Check sheet for the drawn part. Datum: minimum x, y, z corner. Units: mm. A direction names the side the tool comes from. Round coordinates to 2 decimals unless told otherwise and drop trailing zeros. Order: outer loops, then holes, each group sorted by start corner. A loop starts at its lowest first (then second) coordinate and runs counter-clockwise, first axis right, second up. Notation, with made-up numbers: (58, -34) -> (82, -34) arc R33 cw to (82, -5) -> close; hole circle Ø11 at (-2.5, -32). An arc over 180 degrees is marked (long way). Answer in a Markdown table with one row per item.
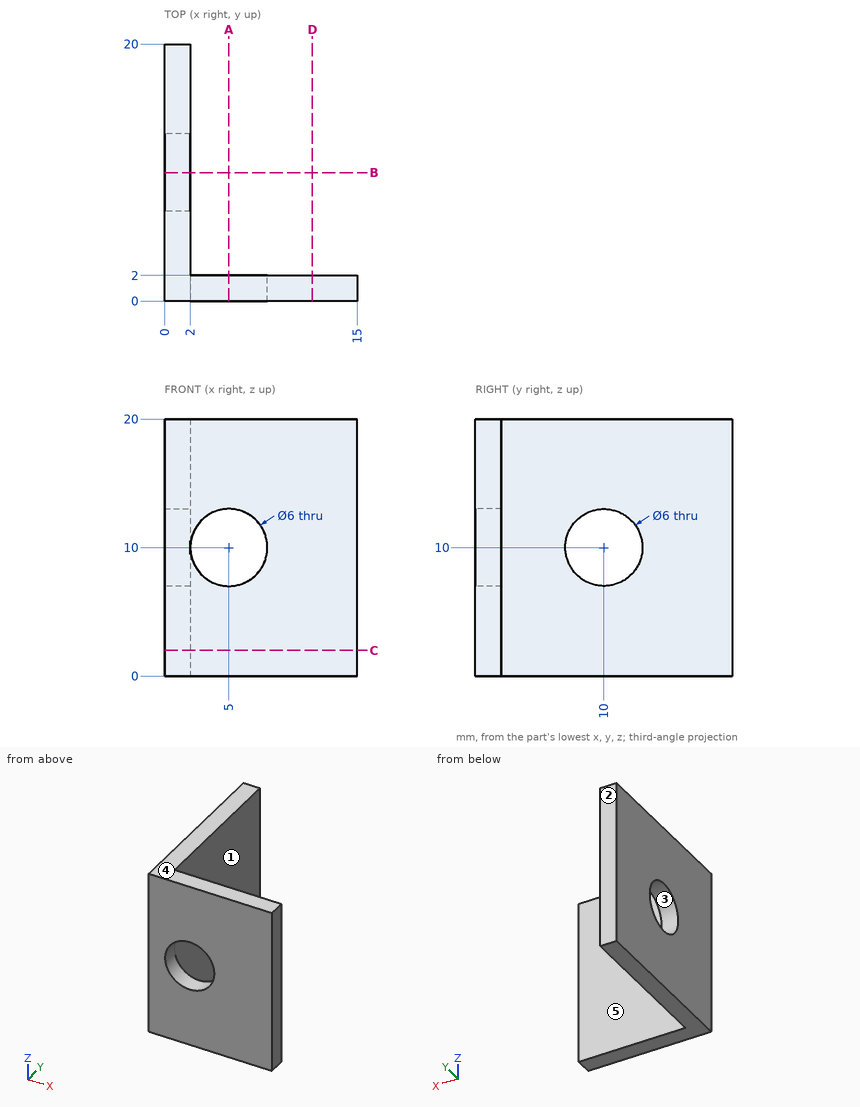
(1) Depth check by flat-ended pin: pin 1 Ø3.5 at (x, z) = (5, 10) entering from +Y; pin 2 Ø8 at (y, z) = (16.5, 12) entering from +X; pin 3 Ø4 at (x, y) = (12.5, 2.5) entering from -Z; pin 4 Ø6.5 at (x, z) = (7.5, 10) entering from +Y. Enter the tip coordinate at first touch or a pass-through.
Solutions:
| item | result |
|---|---|
| pin 1 | through |
| pin 2 | x = 2 |
| pin 3 | z = 0 |
| pin 4 | y = 2 |
(2) Section check C-C on z = 2. Record the boundary of the cut face in (x, y).
Solutions:
| item | result |
|---|---|
| outline | (0, 0) -> (15, 0) -> (15, 2) -> (2, 2) -> (2, 20) -> (0, 20) -> close |
(3) Scan lines: probe 1 along X at (y, z) = (0.5, 10); probe 2 along Z at (x, y) = (5, 1.3). Record each from-to range of solid material in increasing order. Write a range as from..to.
Solutions:
| item | result |
|---|---|
| probe 1 | 0..2, 8..15 |
| probe 2 | 0..7, 13..20 |
(4) Draft check along Y on the marked faces 3, 4 and 5. Enter one of: pulls with the +Y half, pulls with the -Y half, needs draft (parallel to the pull), parting line crosses it, or undercut.
Solutions:
| item | result |
|---|---|
| face 3 | undercut |
| face 4 | needs draft |
| face 5 | pulls with the +Y half |
(5) Section check D-D on x = 11.5. Record the boundary of the cut face in (y, z), plus the area to 3 significant figures.
Solutions:
| item | result |
|---|---|
| outline | (0, 0) -> (2, 0) -> (2, 20) -> (0, 20) -> close |
| area | 40.0 mm^2 |
(6) Section check A-A on x = 5. Record the boundary of the cut face in (y, z).
Solutions:
| item | result |
|---|---|
| outline | (0, 0) -> (2, 0) -> (2, 7) -> (0, 7) -> close; (0, 13) -> (2, 13) -> (2, 20) -> (0, 20) -> close |
(7) Tool access check on the marked faces 1 and 2. Record the directions out of +Z, -Z, +X, -X, +Y, -Y that give a thin tool (end or side, any length) a straight path to the whole face; none if there is none.
Solutions:
| item | result |
|---|---|
| face 1 | +Z, -Z, +X, +Y |
| face 2 | +Z, -Z, +X, -X, +Y |
